Autodesk Inventor part; units mm, degrees
ref_plane "YZ Plane" through (0, 0, 0) normal (1, 0, 0) x (0, 1, 0)
ref_plane "XZ Plane" through (0, 0, 0) normal (0, 1, 0) x (-1, 0, 0)
ref_plane "XY Plane" through (0, 0, 0) normal (0, 0, 1) x (1, 0, 0)
sketch "Sketch1" plane through (0, 0, 0) normal (0, 0, 1) x (1, 0, 0)
  circle A0 centre (4, 4) radius 1.2
  circle A1 centre (4, 4) radius 1.5
  point P0 (0, 0)
  dimension "d0" = 3
extrude "Extrusion1" add sketch "Sketch1" against normal blind 25 contours A0 | A1
sketch "Sketch2" plane through (4, 4, 0) normal (0, 0, 1) x (1, 0, 0)
  circle A0 centre (0, 0) radius 1.5
  circle A1 centre (0, 0) radius 2.8
  point P0 (-4, -4)
  dimension "d3" = 5.6
extrude "Extrusion2" add sketch "Sketch2" along normal blind 3 contours A0 | A1
fillet "Fillet1" radius 0.3 1 edges at (1.2, 4, 3)
sketch "Sketch3" plane through (4, 4, 0) normal (0, 0, -1) x (-1, 0, 0)
  circle A0 centre (0, 0) radius 2.8
  circle A1 centre (0, 0) radius 1.5
  circle A2 centre (0, 0) radius 2.75
  point P0 (4, -4)
  dimension "d7" = 5.5
extrude "Extrusion3" cut sketch "Sketch3" against normal blind 0.5 contours A0
sketch "Sketch4" plane through (4, 4, 3) normal (0, 0, 1) x (1, 0, 0)
  circle A0 centre (0, 0) radius 2.5
  line L0 (0.7217, 1.25) -> (1.4434, 0)
  line L1 (1.4434, 0) -> (0.7217, -1.25)
  line L2 (0.7217, -1.25) -> (-0.7217, -1.25)
  line L3 (-0.7217, -1.25) -> (-1.4434, 0)
  line L4 (-1.4434, 0) -> (-0.7217, 1.25)
  line L5 (-0.7217, 1.25) -> (0.7217, 1.25)
  point P0 (-4, -4)
  dimension "d10" = 2.5
extrude "Extrusion4" cut sketch "Sketch4" against normal blind 2 contours L0 L1 L2 L3 L4 L5
thread "Thread1"
properties part number "m3 6" material "Steel"
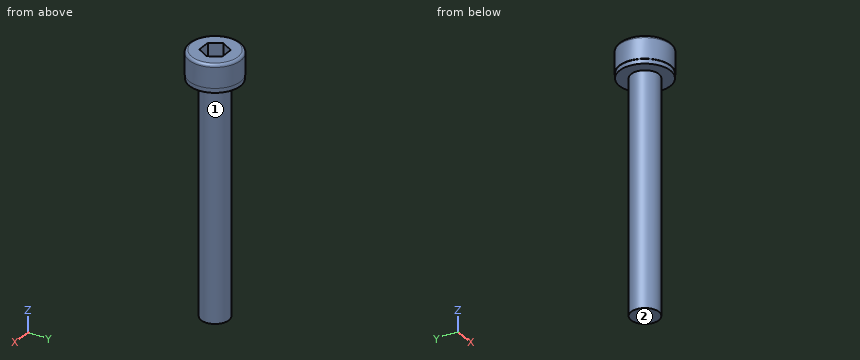
Read the model definition and answer for the solid it produces. Units are mm, in the model's axes. Face numbers are marked on the shaded views. A direction names the side the tool comes from. Coordinates: 2 decimals unless noted, no trailing zeros. Loops run counter-clockwise (first coordinate to the right, second up) from the corner with the lowest first, then second, coordinate; pieces in that order, holes last. Notation, with made-up numbers: (-37.75, 87) - (-8.75, 87) arc R9 cw to (-8.75, 104) - close; hole circle Ø9 at (44.25, 69.5). An arc over 180 degrees is marked (long way). Answer in a Markdown table with one row per item.
Q1. Straight lines are drawn through the part: line 1 along Z through (x, y) = (4.7, 6.1); line 2 along Z through (x, y) = (4.2, 4.5); line 3 along X through (y, z) = (3.9, -4). For each, find the intervals that lie inside material, in ascending order. Write a range as [from, to].
Here are the results:
| item | result |
|---|---|
| line 1 | z = [0, 3] |
| line 2 | z = [-25, 1] |
| line 3 | x = [2.5, 5.5] |
Q2. Find section B-B on z = 0.75. Write down the section's boundary in (x, y).
Here are the results:
| item | result |
|---|---|
| outline | circle Ø5.6 at (4, 4) |
Q3. Given P1, Ø2, axis at y = 4, z = -19, coming from the +X side; P2, Ø1, axis at x = 5.5, z = -13, coming from the +Y side; P3, Ø1.5, axis at y = 5.5, z = -20.5, coming from the +X side, each flat-ended and moving along its own axis, determine where each tip first touches the part or whether it passes through.
Here are the results:
| item | result |
|---|---|
| P1 | stops at x = 5.5 |
| P2 | stops at y = 5.12 |
| P3 | stops at x = 5.3 |
Q4. Find section C-C on z = -8.25. Write down the section's boundary in (x, y), plus the area to 3 significant figures.
Here are the results:
| item | result |
|---|---|
| outline | circle Ø3 at (4, 4) |
| area | 7.07 mm^2 |
Q5. Find section A-A on x = 4. Write down the section's boundary in (y, z), plus the area to 3 significant figures.
Here are the results:
| item | result |
|---|---|
| outline | (1.2, 0.5) - (1.25, 0.5) - (1.25, 0) - (2.5, 0) - (2.5, -25) - (5.5, -25) - (5.5, 0) - (6.75, 0) - (6.75, 0.5) - (6.8, 0.5) - (6.8, 2.7) arc R0.3 ccw to (6.5, 3) - (5.25, 3) - (5.25, 1) - (2.75, 1) - (2.75, 3) - (1.5, 3) arc R0.3 ccw to (1.2, 2.7) - close |
| area | 86.7 mm^2 |
Q6. For the marked faces 1 and 2, determine the directions among +Z, -Z, +X, -X, +Y, -Y from which every point of the face is accessible in a straight line to the end or side of a thin tool.
Here are the results:
| item | result |
|---|---|
| face 1 | -Z |
| face 2 | -Z, +X, -X, +Y, -Y |
